Part model, mm, in its own coordinate system. Face numbers are marked on the shaded views. Round coordinates to 2 decimals unless told otherwise and drop trailing zeros. Write each loop counter-clockwise with the first axis right and the second up, starting at its lowest first coordinate (ties: lowest second). Pieces come first, ordered by that corner, then holes. Notation, with made-up numbers: (64, -10) -> (82, -10) arc R30 ccw to (82, 19) -> close; hole circle Ø10 at (-10, -34.75). An arc over 180 degrees is marked (long way). Return JSON: item names as keys, results as strings. Group by question number.
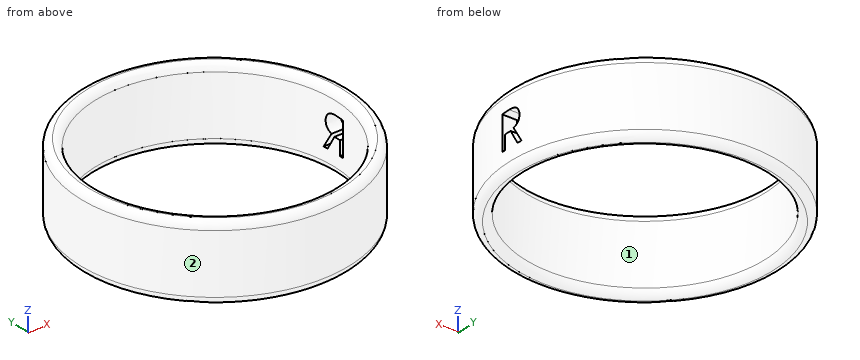
```python
from build123d import *

# Parameters (mm, degrees)
F0_R     = 9
F0_R_2   = 8
F1_DEPTH = 5
F2_R     = 0.49999
F3_R     = 0.49999
F6_DEPTH = 25


# Not quite as in the source:
# - a fillet or chamfer is up to 0.001 mm smaller than in the source, because OpenCascade refuses the exact size


with BuildPart() as f1:
    # F0 (on Top) → F1 (new body)
    with BuildSketch(Plane.XY):
        Circle(F0_R)
        Circle(F0_R_2, mode=Mode.SUBTRACT)
    extrude(amount=F1_DEPTH)

    # F2 (radius 0.5 in the source; OpenCascade refuses exactly that, so slightly less here)
    f2_edges = [f1.edges().sort_by_distance(p)[0] for p in [
        (-8, 0, 5),
        (-9, 0, 5),
    ]]
    fillet(f2_edges, radius=F2_R)

    # F3 (radius 0.5 in the source; OpenCascade refuses exactly that, so slightly less here)
    f3_edges = [f1.edges().sort_by_distance(p)[0] for p in [
        (-8, 0, 0),
        (-9, 0, 0),
    ]]
    fillet(f3_edges, radius=F3_R)

    # F5 (on offset) → F6 (cut)
    with BuildSketch(Plane.YZ.offset(25)):
        with BuildLine():
            Line((-0.5083193487, 1.3498821063), (-0.5083193487, 2.2919357963))
            Line((-0.5083193487, 2.2919357963), (-0.0353092327, 2.2919357963))
            Line((-0.0353092327, 2.2919357963), (0.5130651784, 1.3498821063))
            Line((0.5130651784, 1.3498821063), (0.8244387138, 1.3498821063))
            Line((0.8244387138, 1.3498821063), (0.2091289089, 2.3677959092))
            add(Edge.make_bspline(
                [(0.6647854042, 2.9751726304), (0.6647854042, 2.5259617656), (0.2091289089, 2.3677959092)],
                knots=[0, 0, 0, 1, 1, 1], degree=2))
            add(Edge.make_bspline(
                [(0.465714585, 3.4556200122), (0.6647854042, 3.2959667027), (0.6647854042, 2.9751726304)],
                knots=[0, 0, 0, 1, 1, 1], degree=2))
            add(Edge.make_bspline(
                [(-0.1503389465, 3.6152733218), (0.2666437658, 3.6152733218), (0.465714585, 3.4556200122)],
                knots=[0, 0, 0, 1, 1, 1], degree=2))
            Line((-0.1503389465, 3.6152733218), (-0.7715985641, 3.6152733218))
            Line((-0.7715985641, 3.6152733218), (-0.7715985641, 1.3498821063))
            Line((-0.7715985641, 1.3498821063), (-0.5083193487, 1.3498821063))
        make_face()
        Polygon((-0.5905224825, 2.4278266355), (-0.5905224825, 3.4481487237), (0, 3.4917523153), (0.4821238399, 3.2650141511), (0.4821238399, 2.7940962464), (0.1768992952, 2.4278266355), align=None, mode=Mode.SUBTRACT)
        Polygon((0, 3.4917523153), (-0.5905224825, 3.4481487237), (-0.5905224825, 2.4278266355), (0.1768992952, 2.4278266355), (0.4821238399, 2.7940962464), (0.4821238399, 3.2650141511), align=None)
        with BuildLine():
            Line((-0.1468682223, 2.5180286819), (-0.5083193487, 2.5180286819))
            Line((-0.5083193487, 2.5180286819), (-0.5083193487, 3.3842222589))
            Line((-0.5083193487, 3.3842222589), (-0.1657092961, 3.3842222589))
            add(Edge.make_bspline(
                [(0.2597023175, 3.2850587126), (0.1273189832, 3.3842222589), (-0.1657092961, 3.3842222589)],
                knots=[0, 0, 0, 1, 1, 1], degree=2))
            add(Edge.make_bspline(
                [(0.3920856519, 2.9612897339), (0.3920856519, 3.1858951663), (0.2597023175, 3.2850587126)],
                knots=[0, 0, 0, 1, 1, 1], degree=2))
            add(Edge.make_bspline(
                [(0.2619334973, 2.6288439449), (0.3920856519, 2.7396592079), (0.3920856519, 2.9612897339)],
                knots=[0, 0, 0, 1, 1, 1], degree=2))
            add(Edge.make_bspline(
                [(-0.1468682223, 2.5180286819), (0.1317813428, 2.5180286819), (0.2619334973, 2.6288439449)],
                knots=[0, 0, 0, 1, 1, 1], degree=2))
        make_face(mode=Mode.SUBTRACT)
        with BuildLine():
            Line((-0.5083193487, 3.3842222589), (-0.5083193487, 2.5180286819))
            Line((-0.5083193487, 2.5180286819), (-0.1468682223, 2.5180286819))
            add(Edge.make_bspline(
                [(-0.1468682223, 2.5180286819), (0.1317813428, 2.5180286819), (0.2619334973, 2.6288439449)],
                knots=[0, 0, 0, 1, 1, 1], degree=2))
            add(Edge.make_bspline(
                [(0.2619334973, 2.6288439449), (0.3920856519, 2.7396592079), (0.3920856519, 2.9612897339)],
                knots=[0, 0, 0, 1, 1, 1], degree=2))
            add(Edge.make_bspline(
                [(0.3920856519, 2.9612897339), (0.3920856519, 3.1858951663), (0.2597023175, 3.2850587126)],
                knots=[0, 0, 0, 1, 1, 1], degree=2))
            add(Edge.make_bspline(
                [(0.2597023175, 3.2850587126), (0.1273189832, 3.3842222589), (-0.1657092961, 3.3842222589)],
                knots=[0, 0, 0, 1, 1, 1], degree=2))
            Line((-0.1657092961, 3.3842222589), (-0.5083193487, 3.3842222589))
        make_face()
    extrude(amount=-F6_DEPTH, mode=Mode.SUBTRACT)


solid = f1.part
```
Item 1: Cut at B-B (z = 4). Write the cut outline in (x, y), then the cut area to 3 significant figures.
Item 2: Two-plate mould, pull along Y, no slides. Class the marked faces 1 and 2: released by +Y, released by -Y, zero draft, split by the parting line, or undercut.
Item 3: Flat gauge pins, fed straight in: P1, Ø2, axis at x = -1.5, z = 4, coming from the -Y side; P2, Ø0.5, axis at x = 8.5, z = 1.5, coming from the -Y side; P3, Ø3, axis at y = -4.5, z = 3.5, coming from the -X side. Where does each tip first touch, or does it go through?
Item 4: Wall check: L1, parallel to Y at x = 0, z = 1.95; L2, parallel to Y at x = -1.5, z = 1.65; L3, parallel to X at y = 1, z = 1.15. Give the ranges that are in metal, low to high.
Checks:
{
 "1": {"outline": "circle Ø18 at (0, 0); hole circle Ø16 at (0, 0)", "area": "53.4 mm2"},
 "2": {"face 1": "undercut", "face 2": "split by the parting line"},
 "3": {"P1": "stops at y = -8.99", "P2": "stops at y = -3.6", "P3": "stops at x = -8.49"},
 "4": {"L1": "y = -9 to -8, 8 to 9", "L2": "y = -8.87 to -7.86, 7.86 to 8.87", "L3": "x = -8.94 to -7.94, 7.94 to 8.94"}
}
